Model file for the job. Use its own axes, mm. Face numbers are marked on the shaded views. A direction names the side the tool comes from. Give positions to 0.01 mm unless a question says otherwise; leave off trailing zeros. Loops run counter-clockwise (first coordinate to the right, second up) from the corner with the lowest first, then second, coordinate; pieces in that order, holes last. Notation, with made-up numbers: M 30,25 L 80,25 A10 ccw 80,41 Z; hole C 42.25,-1 d1. An arc over 180 degrees is marked long. Answer in a Markdown table with one row per item.
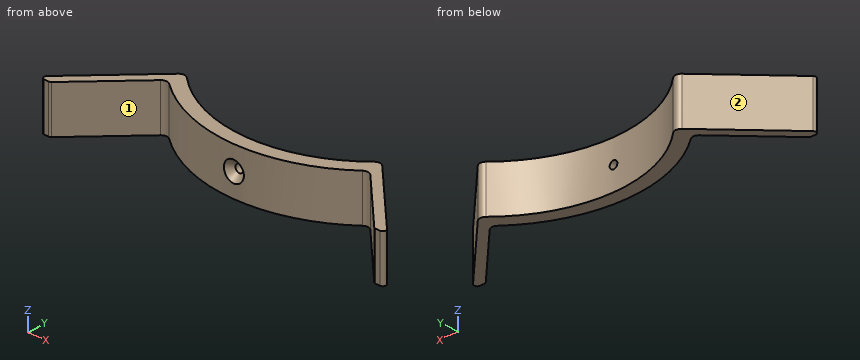
Autodesk Inventor part; units mm, degrees
ref_plane "YZ Plane" through (0, 0, 0) normal (1, 0, 0) x (0, 1, 0)
ref_plane "XZ Plane" through (0, 0, 0) normal (0, 1, 0) x (-1, 0, 0)
ref_plane "XY Plane" through (0, 0, 0) normal (0, 0, 1) x (1, 0, 0)
sketch "Sketch1" plane through (0, 0, 0) normal (0, 0, 1) x (1, 0, 0)
  circle A0 centre (0, 0) radius 45
  line L0 (0, 0) -> (0, -60)
  line L1 (0, -60) -> (60, -60)
  line L2 (60, -60) -> (31.8198, -31.8198)
  line L3 (0, -60) -> (-60, -60)
  line L4 (-60, -60) -> (-31.8198, -31.8198)
  line L5 (29.6985, -33.9411) -> (52.7574, -57)
  line L6 (52.7574, -57) -> (0, -57)
  line L7 (-29.6985, -33.9411) -> (-52.7574, -57)
  line L8 (-52.7574, -57) -> (0, -57)
  circle A1 centre (0, 0) radius 49.5
  line L9 (-52.7574, -57) -> (-57, -57)
  line L10 (52.7574, -57) -> (57, -57)
  point P0 (0, -45)
  point P1 (32.8161, -37.0588)
  point P2 (-32.8161, -37.0588)
  dimension "d0" = 90
  dimension "d1" = 60
  dimension "d2" = 60
  dimension "d3" = 45
  dimension "d18" = 3
  dimension "d19" = 3
  dimension "d20" = 4.5
extrude "Extrusion1" add sketch "Sketch1" along normal blind 15 contours A0 L0 A1 L4 | L2 A1 L0 A0 | A1 L7 L9 L4 | L2 L10 L5 A1
sketch "Sketch7" plane through (-60, -57, 0) normal (0, -1, 0) x (1, 0, 0)
  circle A0 centre (60, 7.5) radius 3.5
  circle A1 centre (60, 7.5) radius 1.25
  point P0 (60, 0)
  dimension "d31" = 2.5
extrude "Extrusion7" cut sketch "Sketch7" against normal blind 21.25 contours A1
chamfer "Chamfer1" distance 2 angle 45 1 edges at (-1.25, -49.4842, 7.5043)
fillet "Fillet1" radius 2 4 edges at (-32.8161, -37.0588, 7.5) (32.8161, -37.0588, 7.5) (-31.8198, -31.8198, 7.5) (31.8198, -31.8198, 7.5)
fillet "Fillet3" radius 1 4 edges at (-52.7574, -57, 7.5) (-57, -57, 7.5) (57, -57, 7.5) (52.7574, -57, 7.5)
properties part number "Horizontal Base_3DPrint"
(1) Which spindle directions (+Z, -Z, +X, -X, +Y, -Y) get a long thin tool onto all of the face, cutting with end or side? Do the marked faces 1 and 2. Say none if no direction does.
Established:
| item | result |
|---|---|
| face 1 | +Z, -Z, -Y |
| face 2 | +Z, -Z, -X, +Y |
(2) Saw through at C-C, the plane y = -42.75. Give the cut face in (x, z).
Established:
| item | result |
|---|---|
| outline | M -42.75,0 L -38.51,0 L -38.51,15 L -42.75,15 Z; M -24.95,0 L -14.05,0 L -14.05,15 L -24.95,15 Z; M 14.05,0 L 24.95,0 L 24.95,15 L 14.05,15 Z; M 38.51,0 L 42.75,0 L 42.75,15 L 38.51,15 Z |
(3) Saw through at B-B, the plane y = -54.25. Give the cut face in (x, z), and give its area (3 significant figures).
Established:
| item | result |
|---|---|
| outline | M -54.25,0 L -50.01,0 L -50.01,15 L -54.25,15 Z; M 50.01,0 L 54.25,0 L 54.25,15 L 50.01,15 Z |
| area | 127 mm2 |
(4) Wall check: L1, parallel to X at y = -39.5, z = 10; L2, parallel to Z at x = 0, y = -45.75; L3, parallel to X at y = -54, z = 6. Give the ranges that are in metal, low to high.
Established:
| item | result |
|---|---|
| L1 | x = -39.5 to -35.26, -29.83 to -21.56, 21.56 to 29.83, 35.26 to 39.5 |
| L2 | z = 0 to 6.25, 8.75 to 15 |
| L3 | x = -54 to -49.76, 49.76 to 54 |
(5) Saw through at D-D, the plane x = -46. Give the cut face in (y, z).
Established:
| item | result |
|---|---|
| outline | M -50.24,0 L -46,0 L -46,15 L -50.24,15 Z |
(6) Flat gauge pins, fed straight in: P1, Ø6, axis at y = -45.5, z = 6.5, coming from the +X side; P2, Ø5, axis at y = -42.5, z = 13.5, coming from the -X side; P3, Ø2, axis at y = -46.5, z = 12.5, coming from the -X side. Where does each tip first touch, or does it go through?
Established:
| item | result |
|---|---|
| P1 | stops at x = 48.5 |
| P2 | stops at x = -45 |
| P3 | stops at x = -47.5 |
(7) Saw through at A-A, the plane z = 12.25. Give the cut face in (x, y).
Established:
| item | result |
|---|---|
| outline | M -55.29,-55.29 A1 ccw -54.59,-57 L -53.17,-57 A1 ccw -52.46,-56.71 L -34.12,-38.37 A2 cw -31.44,-38.23 A49.5 ccw 31.44,-38.23 A2 cw 34.12,-38.37 L 52.46,-56.71 A1 ccw 53.17,-57 L 54.59,-57 A1 ccw 55.29,-55.29 L 33.2,-33.2 A2 ccw 30.44,-33.15 A45 cw -30.44,-33.15 A2 ccw -33.2,-33.2 Z |
